```python
from build123d import *

# Parameters (mm, degrees)
CROQUIS1_W                 = 2.4
CROQUIS1_H                 = 22.9
CROQUIS3_R                 = 1.5
CORTAR_EXTRUIR1_DEPTH      = 9
CORTAR_EXTRUIR2_DEPTH      = 12.7
CORTAR_EXTRUIR2_DEPTH_BACK = 14
CROQUIS5_W                 = 0.4
CROQUIS5_H                 = 7.15
CORTAR_EXTRUIR3_DEPTH      = 9.7
CORTAR_EXTRUIR3_DEPTH_BACK = 14
CROQUIS6_W                 = 7.15
CROQUIS6_H                 = 0.4


# Read off the part's stored shape, not the designer's step: #8-32 Roscas Standard Taladro2
with BuildPart() as part:
    # Croquis1 → Revolución1 (revolve)
    with BuildSketch(Plane(origin=(0, 0, 0), x_dir=(1, 0, 0), z_dir=(0, 1, 0))):
        with Locations((1.2, 11.45)):
            Rectangle(CROQUIS1_W, CROQUIS1_H)
    revolve(axis=Axis((0, 0, 0), (0, 0, -1)))

    # Croquis2 → Revolución2 (revolve)
    with BuildSketch(Plane(origin=(0, 0, 0), x_dir=(1, 0, 0), z_dir=(0, 1, 0)), mode=Mode.PRIVATE) as revoluci_n2_sk:
        Polygon((-4.2, 0), (-2.4, 0), (-2.4, 7.15), align=None)
    revolve(revoluci_n2_sk.sketch.rotate(Axis((0, 0, 0), (0, 0, -1)), 180), axis=Axis((0, 0, 0), (0, 0, -1)))

    # Croquis3 → Cortar-Extruir1 (cut)
    with BuildSketch(Plane.XY):
        Circle(CROQUIS3_R)
    extrude(amount=-CORTAR_EXTRUIR1_DEPTH, mode=Mode.SUBTRACT)

    # Croquis5 → Cortar-Extruir2 (cut, two sides: drawn at the far end of the back side and taken through both)
    with BuildSketch(Plane(origin=(0, 0, 0), x_dir=(1, 0, 0), z_dir=(0, 1, 0)).offset(-CORTAR_EXTRUIR2_DEPTH_BACK)):
        with Locations((0, 3.575)):
            Rectangle(CROQUIS5_W, CROQUIS5_H)
    extrude(amount=CORTAR_EXTRUIR2_DEPTH + CORTAR_EXTRUIR2_DEPTH_BACK, mode=Mode.SUBTRACT)

    # Croquis6 → Cortar-Extruir3 (cut, two sides: drawn at the far end of the back side and taken through both)
    with BuildSketch(Plane(origin=(0, 0, 0), x_dir=(0, 0, -1), z_dir=(1, 0, 0)).offset(-CORTAR_EXTRUIR3_DEPTH_BACK)):
        with Locations((3.575, 0)):
            Rectangle(CROQUIS6_W, CROQUIS6_H)
    extrude(amount=CORTAR_EXTRUIR3_DEPTH + CORTAR_EXTRUIR3_DEPTH_BACK, mode=Mode.SUBTRACT)

    # #8-32 Roscas Standard Taladro2 outline → #8-32 Roscas Standard Taladro2 (revolve, cut)
    with BuildSketch(Plane.XZ):
        Polygon((1.61036, -22.9), (2.4, -22.9), (2.4, -9.4), (2.0828, -9.4), (2.0828, -22.42756), align=None)
    revolve(axis=Axis((0, 0, 0), (0, 0, 1)), mode=Mode.SUBTRACT)


solid = part.part
```
Model file for the job. Use its own axes, mm. A direction names the side the tool comes from. Coordinates: 2 decimals unless noted, no trailing zeros. Order: outer loops, then holes, each group sorted by start corner. A loop starts at its lowest first (then second) coordinate and runs counter-clockwise, first axis right, second up. Notation, with made-up numbers: M 20,78.5 L 46,78.5 A30 cw 46,102.5 Z; hole C 70,-39 d8. An arc over 180 degrees is marked long. Answer as CSV lines item,"result".
(1) Flat gauge pins, fed straight in: pin 1 (3 mm diameter, centred on x = 2.5, z = -7.5, fed in from -Y); pin 2 (1.5 mm diameter, centred on x = 2.5, z = -13.5, fed in from +Y); pin 3 (0.8 mm diameter, centred on x = 3, z = -3.5, fed in from +Y). Where does each tip first touch, or does it go through?
Geometry says:
pin 1,"stops at y = -2.19"
pin 2,"stops at y = 1.13"
pin 3,"stops at y = 2.09"
(2) Pull direction Y, two halves, no side cores. Call faces 1 (the conical face through (2.366, -2.318, -3.525)), 2 (the flat face through (0, 0, -9)), 3 (the flat face through (0.2, -3, -3)): +Y half, -Y half, draft (parallel to the pull), parting line (faces both ways), or undercut.
Geometry says:
face 1,"-Y half"
face 2,"undercut"
face 3,"draft"
(3) Band-saw the part on B-B, the plane z = -12.5. List the corners of the cut face in (x, y).
Geometry says:
outline,"C 0,0 d4.17"
(4) Wall check: line 1 along Z through (x, y) = (-0.5, -0.25); line 2 along Y through (x, z) = (-2.5, -4.5); line 3 along X through (y, z) = (2.75, -3.25). Give the ranges that are in metal, low to high.
Geometry says:
line 1,"z = -22.9 to -9"
line 2,"y = -1.78 to -0.2, 0.2 to 1.78"
line 3,"x = -1.97 to -0.2, 0.2 to 1.97"
(5) 3-axis set-ups, long thin cutter, end or side, ignore diameter. For faces 4 (the flat face through (-3, -0.2, -3)), 5 (the flat face through (0.2, 3, -3)), 6 (the flat face through (-1, 2, -9.4)): which of +Z, -Z, +X, -X, +Y, -Y reach the whole face in a straight line?
Geometry says:
face 4,"+Z, +X, -X"
face 5,"+Z, +Y, -Y"
face 6,"-Z"
(6) Band-saw the part on A-A, the plane z = -3.5. List the corners of the cut face in (x, y).
Geometry says:
outline,"M -3.31,-0.2 A3.32 ccw -0.2,-3.31 L -0.2,-1.49 A1.5 cw -1.49,-0.2 Z; M -3.31,0.2 L -1.49,0.2 A1.5 cw -0.2,1.49 L -0.2,3.31 A3.32 ccw Z; M 0.2,-3.31 A3.32 ccw 3.31,-0.2 L 1.49,-0.2 A1.5 cw 0.2,-1.49 Z; M 0.2,1.49 A1.5 cw 1.49,0.2 L 3.31,0.2 A3.32 ccw 0.2,3.31 Z"
